Geometry check sheet. Reference: the model listing, model coordinates, mm. A direction names the side the tool comes from. Round coordinates to 2 decimals unless told otherwise and drop trailing zeros. Loops run counter-clockwise (first coordinate to the right, second up) from the corner with the lowest first, then second, coordinate; pieces in that order, holes last. Notation, with made-up numbers: (15, 78.5) - (22, 78.5) arc R8 cw to (22, 82.5) - close; hole circle Ø3 at (5, 28.25). An arc over 180 degrees is marked (long way). Answer in a Markdown table with one row per item. Add a question column.
```python
from build123d import *

# Parameters (mm, degrees)
ESQUISSE1_W             = 107
ESQUISSE1_H             = 29
BOSS_EXTRU_1_DEPTH      = 14
ESQUISSE2_W             = 79
ESQUISSE2_H             = 19
ENL_V_MAT_EXTRU_1_DEPTH = 58.170796741
CONG_1_R                = 5
ESQUISSE3_R             = 1.5
ENL_V_MAT_EXTRU_2_DEPTH = 5


with BuildPart() as part:
    # Esquisse1 → Boss.-Extru.1 (new body)
    with BuildSketch(Plane.XY):
        Rectangle(ESQUISSE1_W, ESQUISSE1_H)
    extrude(amount=BOSS_EXTRU_1_DEPTH)

    # Esquisse2 → Enlèv. mat.-Extru.1 (cut, through all)
    with BuildSketch(Plane.XY.offset(14)):
        with Locations((0, -5)):
            Rectangle(ESQUISSE2_W, ESQUISSE2_H)
    extrude(amount=-ENL_V_MAT_EXTRU_1_DEPTH, mode=Mode.SUBTRACT)

    # Congé1
    cong_1_edges = [part.edges().sort_by_distance(p)[0] for p in [
        (-53.5, 0, 14),
        (39.5, -5, 0),
        (39.5, 4.5, 7),
        (-39.5, -5, 0),
        (0, 4.5, 0),
        (-39.5, 4.5, 7),
        (39.5, -5, 14),
        (0, 4.5, 14),
        (-39.5, -5, 14),
        (53.5, 0, 14),
        (-53.5, 0, 0),
        (0, 14.5, 0),
        (53.5, 0, 0),
        (-53.5, 14.5, 7),
        (53.5, 14.5, 7),
        (0, 14.5, 14),
    ]]
    fillet(cong_1_edges, radius=CONG_1_R - 0.0001)  # a hair under: the kernel refuses the full size

    # Esquisse3 → Enlèv. mat.-Extru.2 (cut)
    with BuildSketch(Plane.XZ.offset(14.5)):
        with Locations(Location((-46.5, 7, 0), (0, 0, 270))):
            Circle(ESQUISSE3_R)
        with Locations(Location((46.5, 7, 0), (0, 0, 270))):
            Circle(ESQUISSE3_R)
    extrude(amount=-ENL_V_MAT_EXTRU_2_DEPTH, mode=Mode.SUBTRACT)


solid = part.part
```
Q1. Cross-section at C-C, the plane x = -46.5. Enter the section's corners in (y, z), plus the area to 3 significant figures.
Q2. Set-up check for faces 1 (the flat face through (-46, -9.5, 7)), 2 (the cylindrical face through (0.48, 6, 12.57)), 3 (the cylindrical face through (38.07, 3, 6.97)): record each of +Z, -Z, +X, -X, +Y, -Y from which the full face is reachable in a straight line by a thin tool's end or side.
Q3. Cross-section at A-A, the plane y = -3.25. Enter the section's corners in (x, z), plus the area to 3 significant figures.
Q4. Depth check by flat-ended pin: P1, Ø2, axis at x = 37.5, y = -7, coming from the -Z side; P2, Ø3, axis at x = -12, z = 8, coming from the -Y side; P3, Ø3.5, axis at x = 47, z = 7, coming from the -Y side; P4, Ø2.5, axis at x = -46.5, z = 7, coming from the -Y side. Enter the tip coordinate at first touch or a pass-through.
Q5. Cross-section at B-B, the plane z = 7. Enter the section's corners in (x, y).
Q6. Release check for a two-part mould opening along X. For faces 4 (the cylindrical face through (45, -12, 7)), 5 (the flat face through (53.5, -3, 7)), 6 (the flat face through (-39.74, 8.22, 14)) record: +X half, -X half, draft (parallel to the pull), parting line (faces both ways), or undercut.
Q7. Cross-section at D-D, the plane y = 11.75. Enter the section's corners in (x, z).
Q8. Scan lines: line 1 (X direction, y = -12, z = 7); line 2 (X direction, y = -13.5, z = 6.25); line 3 (Y direction, x = 34, z = 6.75). Record each from-to range of solid material in increasing order. Write a range as from..to.
Check sheet entries:
| question | item | result |
|---|---|---|
| 1 | outline | (-14.5, 0) - (9.5, 0) arc R5 ccw to (14.5, 5) - (14.5, 9) arc R5 ccw to (9.5, 14) - (-14.5, 14) - (-14.5, 8.5) - (-9.5, 8.5) - (-9.5, 5.5) - (-14.5, 5.5) - close |
| 1 | area | 380 mm² |
| 2 | face 1 | -Y |
| 2 | face 2 | +Z, -Y |
| 2 | face 3 | +Z, -Z, -Y |
| 3 | outline | (-53.5, 5) arc R5 ccw to (-48.5, 0) - (-44.5, 0) arc R5 ccw to (-39.5, 5) - (-39.5, 9) arc R5 ccw to (-44.5, 14) - (-48.5, 14) arc R5 ccw to (-53.5, 9) - close; (39.5, 5) arc R5 ccw to (44.5, 0) - (48.5, 0) arc R5 ccw to (53.5, 5) - (53.5, 9) arc R5 ccw to (48.5, 14) - (44.5, 14) arc R5 ccw to (39.5, 9) - close |
| 3 | area | 349 mm² |
| 4 | P1 | through |
| 4 | P2 | y = 4.5 |
| 4 | P3 | y = -14.5 |
| 4 | P4 | y = -9.5 |
| 5 | outline | (-53.5, -14.5) - (-48, -14.5) - (-48, -9.5) - (-45, -9.5) - (-45, -14.5) - (-39.5, -14.5) - (-39.5, -0.5) arc R5 cw to (-34.5, 4.5) - (34.5, 4.5) arc R5 cw to (39.5, -0.5) - (39.5, -14.5) - (45, -14.5) - (45, -9.5) - (48, -9.5) - (48, -14.5) - (53.5, -14.5) - (53.5, 9.5) arc R5 ccw to (48.5, 14.5) - (-48.5, 14.5) arc R5 ccw to (-53.5, 9.5) - close |
| 6 | face 4 | undercut |
| 6 | face 5 | +X half |
| 6 | face 6 | draft |
| 7 | outline | (-52.97, 5) arc R4.47 ccw to (-48.5, 0.53) - (48.5, 0.53) arc R4.47 ccw to (52.97, 5) - (52.97, 9) arc R4.47 ccw to (48.5, 13.47) - (-48.5, 13.47) arc R4.47 ccw to (-52.97, 9) - close |
| 8 | line 1 | -53.5..-48, -45..-39.5, 39.5..45, 48..53.5 |
| 8 | line 2 | -53.5..-47.8, -45.2..-39.5, 39.5..45.2, 47.8..53.5 |
| 8 | line 3 | 4.5..14.5 |
